Input: part model. Units: mm. Frame: model coordinates. A direction names the side the tool comes from. Give positions to 0.01 mm unless a question says otherwise; leave off trailing zeros. Write each loop counter-clockwise with the first axis right and the second up, starting at its lowest first coordinate (ties: lowest second). Pieces come first, ordered by that corner, then holes.
```python
from build123d import *

# Parameters (mm, degrees)
SKETCH1_W           = 635
SKETCH1_H           = 101.6
BOSS_EXTRUDE1_DEPTH = 12.7
CUT_EXTRUDE1_DEPTH  = 322.789030267
SKETCH3_R           = 9.525
CUT_EXTRUDE2_DEPTH  = 322.789030267


with BuildPart() as part:
    # Sketch1 → Boss-Extrude1 (new body)
    with BuildSketch(Plane(origin=(0, 0, 0), x_dir=(1, 0, 0), z_dir=(0, 1, 0))):
        Rectangle(SKETCH1_W, SKETCH1_H)
    extrude(amount=BOSS_EXTRUDE1_DEPTH)

    # Sketch2 → Cut-Extrude1 (cut, through all)
    with BuildSketch(Plane(origin=(0, 12.7, 0), x_dir=(1, 0, 0), z_dir=(0, 1, 0))):
        with BuildLine():
            Line((-292.1, 12.7), (-317.5, 12.7))
            Line((-317.5, 12.7), (-317.5, 50.8))
            Line((-317.5, 50.8), (-254, 50.8))
            ThreePointArc((-254, 50.8), (-265.159231637, 23.859231637), (-292.1, 12.7))
        make_face()
    cut_extrude1 = extrude(amount=-CUT_EXTRUDE1_DEPTH, mode=Mode.SUBTRACT)

    # Mirror1: Cut-Extrude1 across plane
    add(cut_extrude1.mirror(Plane(origin=(0, 0, 0), x_dir=(0, 0, 1), z_dir=(1, 0, 0))), mode=Mode.SUBTRACT)

    # Sketch3 → Cut-Extrude2 (cut, through all)
    with BuildSketch(Plane(origin=(0, 12.7, 0), x_dir=(1, 0, 0), z_dir=(0, 1, 0))):
        with Locations(Location((0, 28.575, 0), (0, 0, 270))):
            Circle(SKETCH3_R)
    extrude(amount=-CUT_EXTRUDE2_DEPTH, mode=Mode.SUBTRACT)


solid = part.part
```
Item 1: Pin query (flat end, axial travel): pin 1 (6.5 mm diameter, centred on x = -307, y = 9, fed in from -Z). Return the tip coordinate at first contact, or that it passes through.
Item 2: Ray query, line 1 (X direction, y = 3, z = -32.5); line 2 (X direction, y = 1.75, z = -32); line 3 (X direction, y = 1.5, z = -42.5). Return the intervals inside material, ascending.
Item 3: Set-up query: faces 4 (the flat face through (305, 6, -12.7)), 5 (the flat face through (-4, 6, -50.8)), 6 (the flat face through (-305, 6, -12.7)). Return all of +Z, -Z, +X, -X, +Y, -Y with unobstructed straight access to the full face (end or side cutting, diameter ignored); none if empty.
Item 4: Section B-B (y = 3.5). Return loops of the section in (x, z) (3 decimals), and give its area (3 significant figures).
Item 5: Mould query, pull axis X, two halves, no side actions, for faces 1 (the flat face through (-4, 0, -1)), 2 (the flat face through (-317.5, 6, 19)), 3 (the cylindrical face through (2.86, 6.44, -19.49)). Classes: +X half, -X half, draft (parallel to the pull), parting line (faces both ways), or undercut.
Item 6: Section A-A (x = 0). Return loops of the section in (y, z), and give its area (3 significant figures).
Solved:
1. pin 1: stops at z = -12.7
2. line 1: x = -258.68 to -8.68, 8.68 to 258.68
2. line 2: x = -258.96 to -8.89, 8.89 to 258.96
2. line 3: x = -254.92 to 254.92
3. face 4: -Z, +X, +Y, -Y
3. face 5: -Z, +X, -X, +Y, -Y
3. face 6: -Z, -X, +Y, -Y
4. outline: (-317.5, -12.7) - (-292.1, -12.7) arc R38.1 cw to (-254, -50.8) - (254, -50.8) arc R38.1 cw to (292.1, -12.7) - (317.5, -12.7) - (317.5, 50.8) - (-317.5, 50.8) - close; hole circle Ø19.05 at (0, -28.575)
4. area: 60,000 mm2
5. face 1: draft
5. face 2: -X half
5. face 3: undercut
6. outline: (0, -50.8) - (12.7, -50.8) - (12.7, -38.1) - (0, -38.1) - close; (0, -19.05) - (12.7, -19.05) - (12.7, 50.8) - (0, 50.8) - close
6. area: 1,050 mm2
